from build123d import *

# Parameters (mm, degrees)
SKETCH_1_W               = 38
SKETCH_1_H               = 29
EXTRUDE_1_DEPTH          = 2
SKETCH_2_W               = 2
SKETCH_2_H               = 36
EXTRUDE_2_DEPTH          = 7.5
SKETCH_3_R               = 5
SKETCH_3_R_2             = 1.25
CUT_EXTRUDE_1_DEPTH      = 8.5
CUT_EXTRUDE_1_DEPTH_BACK = 3
SKETCH_4_R               = 1.3
CUT_EXTRUDE_2_DEPTH      = 39
CUT_EXTRUDE_3_DEPTH      = 39
FILLET_1_R               = 2
FILLET_3_R               = 0.5
FILLET_4_R               = 2


with BuildPart() as part:
    # 스케치1 → 보스-돌출1 (new body)
    with BuildSketch(Plane(origin=(0, 0, 0), x_dir=(1, 0, 0), z_dir=(0, 1, 0))):
        with Locations((19, 14.5)):
            Rectangle(SKETCH_1_W, SKETCH_1_H)
    extrude(amount=EXTRUDE_1_DEPTH)

    # 스케치2 → 보스-돌출2 (add)
    with BuildSketch(Plane(origin=(0, 2, 0), x_dir=(1, 0, 0), z_dir=(0, 1, 0))):
        with Locations((1, 18)):
            Rectangle(SKETCH_2_W, SKETCH_2_H)
        with Locations((37, 18)):
            Rectangle(SKETCH_2_W, SKETCH_2_H)
    extrude(amount=EXTRUDE_2_DEPTH)

    # 스케치3 → 컷-돌출1 (cut, two sides)
    with BuildSketch(Plane(origin=(0, 2, 0), x_dir=(1, 0, 0), z_dir=(0, 1, 0))) as cut_extrude_1_sk:
        with Locations((19, 14.5)):
            Circle(SKETCH_3_R)
        with Locations((19, 25.5)):
            Circle(SKETCH_3_R_2)
        with Locations((26.778174593, 22.278174593)):
            Circle(SKETCH_3_R_2)
        with Locations((30, 14.5)):
            Circle(SKETCH_3_R_2)
        with Locations((26.778174593, 6.721825407)):
            Circle(SKETCH_3_R_2)
        with Locations((19, 3.5)):
            Circle(SKETCH_3_R_2)
        with Locations((11.221825407, 6.721825407)):
            Circle(SKETCH_3_R_2)
        with Locations((8, 14.5)):
            Circle(SKETCH_3_R_2)
        with Locations((11.221825407, 22.278174593)):
            Circle(SKETCH_3_R_2)
        with Locations((13, 25.5)):
            Circle(SKETCH_3_R_2)
        with Locations((25, 25.5)):
            Circle(SKETCH_3_R_2)
        with Locations((30, 20.5)):
            Circle(SKETCH_3_R_2)
        with Locations((30, 8.5)):
            Circle(SKETCH_3_R_2)
        with Locations((25, 3.5)):
            Circle(SKETCH_3_R_2)
        with Locations((13, 3.5)):
            Circle(SKETCH_3_R_2)
        with Locations((8, 8.5)):
            Circle(SKETCH_3_R_2)
        with Locations((8, 20.5)):
            Circle(SKETCH_3_R_2)
        with Locations((15.5, 22.278174593)):
            Circle(SKETCH_3_R_2)
        with Locations((22.5, 22.278174593)):
            Circle(SKETCH_3_R_2)
        with Locations((26.778174593, 18)):
            Circle(SKETCH_3_R_2)
        with Locations((26.778174593, 11)):
            Circle(SKETCH_3_R_2)
        with Locations((22.5, 6.721825407)):
            Circle(SKETCH_3_R_2)
        with Locations((15.5, 6.721825407)):
            Circle(SKETCH_3_R_2)
        with Locations((11.221825407, 11)):
            Circle(SKETCH_3_R_2)
        with Locations((11.221825407, 18)):
            Circle(SKETCH_3_R_2)
    extrude(amount=CUT_EXTRUDE_1_DEPTH, mode=Mode.SUBTRACT)
    extrude(cut_extrude_1_sk.sketch, amount=-CUT_EXTRUDE_1_DEPTH_BACK, mode=Mode.SUBTRACT)

    # 스케치4 → 컷-돌출2 (cut, through all)
    with BuildSketch(Plane(origin=(38, 0, 0), x_dir=(0, 0, -1), z_dir=(1, 0, 0))):
        with Locations((3.5, 6.7)):
            Circle(SKETCH_4_R)
        with Locations((25.5, 6.7)):
            Circle(SKETCH_4_R)
        with Locations((10.5, 6.7)):
            Circle(SKETCH_4_R)
        with Locations((32.5, 6.7)):
            Circle(SKETCH_4_R)
    extrude(amount=-CUT_EXTRUDE_2_DEPTH, mode=Mode.SUBTRACT)

    # 스케치5 → 컷-돌출3 (cut, through all)
    with BuildSketch(Plane(origin=(38, 0, 0), x_dir=(0, 0, -1), z_dir=(1, 0, 0))):
        Polygon((36, 3.77094162), (29, 2), (36, 2), align=None)
        Polygon((29, 2), (28.116343093, 0), (29, 0), align=None)
    extrude(amount=-CUT_EXTRUDE_3_DEPTH, mode=Mode.SUBTRACT)

    # 필렛1
    fillet_1_edges = [part.edges().sort_by_distance(p)[0] for p in [
        (1, 9.5, -36),
        (1, 9.5, 0),
        (37, 3.77094162, -36),
        (37, 9.5, 0),
        (37, 9.5, -36),
    ]]
    fillet(fillet_1_edges, radius=FILLET_1_R)

    # 필렛3
    fillet_3_edges = [part.edges().sort_by_distance(p)[0] for p in [
        (2, 2, -14.5),
        (36, 2, -14.5),
    ]]
    fillet(fillet_3_edges, radius=FILLET_3_R)

    # 필렛4
    fillet_4_edges = [part.edges().sort_by_distance(p)[0] for p in [
        (0, 0, -14.058171546),
        (38, 0, -14.058171546),
    ]]
    fillet(fillet_4_edges, radius=FILLET_4_R)


solid = part.part
CAD build for the part. Positions are in the model's coordinates, mm. A direction names the side the tool comes from. Round coordinates to 2 decimals unless told otherwise and drop trailing zeros. Write each loop counter-clockwise with the first axis right and the second up, starting at its lowest first coordinate (ties: lowest second). Pieces come first, ordered by that corner, then holes.
(1) Drop flat-ended pins along their axis: P1, Ø3, axis at x = 14, z = -22, coming from the +Y side; P2, Ø1.5, axis at x = 26.78, z = -22.28, coming from the +Y side; P3, Ø8, axis at x = 33.5, z = -15.5, coming from the +Y side. Give the stop position or say it passes through.
(2) Slice it at C-C, the plane x = 30. Write the cut outline in (y, z).
(3) 3-axis set-ups, long thin cutter, end or side, ignore diameter. For faces 4 (the face through (36.986, 4.085, -35.567)), 5 (the face through (37.014, 5.547, -11.1)): which of +Z, -Z, +X, -X, +Y, -Y reach the whole face in a straight line?
(4) Slice it at A-A, the plane x = 13. Write the cut outline in (y, z).
(5) Probe line 1 along X through (y, z) = (5.5, -17.5); line 2 along X through (y, z) = (1.4, -11); line 3 along X through (y, z) = (1.75, -22). List the from-to ranges inside material, lowest first.
(6) Slice it at D-D, the plane z = -20. Write the cut outline in (x, y), and give its area (3 significant figures).
(7) Mould opens along Z. For faces 1 (the face through (27.45, 1.014, -12.054)), 2 (the face through (15, 2, -18)), 3 (the face through (19.266, 1.014, -28.564)) say: pulls with the +Z half, pulls with the -Z half, needs draft (parallel to the pull), parting line crosses it, or undercut.
(8) Slice it at B-B, the plane z = -25.5. Count the separate pieces of the cut face and the enclosed holes in it, and give its area (3 significant figures).
From the geometry:
1. P1: stops at y = 2
1. P2: passes through
1. P3: stops at y = 9.5
2. outline: (0, -28.12) - (2, -29) - (2, -21.75) - (0, -21.75) - close; (0, -19.25) - (2, -19.25) - (2, -15.75) - (0, -15.75) - close; (0, -13.25) - (2, -13.25) - (2, -9.75) - (0, -9.75) - close; (0, -7.25) - (2, -7.25) - (2, 0) - (0, 0) - close
3. face 4: -Z, +X, -Y
3. face 5: +X, -X
4. outline: (0, -28.12) - (2, -29) - (2, -26.75) - (0, -26.75) - close; (0, -24.25) - (2, -24.25) - (2, -4.75) - (0, -4.75) - close; (0, -2.25) - (2, -2.25) - (2, 0) - (0, 0) - close
5. line 1: x = 0 to 2, 36 to 38
5. line 2: x = 0.09 to 9.97, 12.47 to 15.43, 22.57 to 25.53, 28.03 to 37.91
5. line 3: x = 0.02 to 10, 12.44 to 14.28, 16.72 to 21.28, 23.72 to 25.56, 28 to 37.98
6. outline: (0, 2) arc R2 ccw to (2, 0) - (6.85, 0) - (6.85, 2) - (2.5, 2) arc R0.5 cw to (2, 2.5) - (2, 9.5) - (0, 9.5) - close; (9.15, 0) - (28.85, 0) - (28.85, 2) - (9.15, 2) - close; (31.15, 0) - (36, 0) arc R2 ccw to (38, 2) - (38, 9.5) - (36, 9.5) - (36, 2.5) arc R0.5 cw to (35.5, 2) - (31.15, 2) - close
6. area: 95.2 mm2
7. face 1: undercut
7. face 2: needs draft
7. face 3: pulls with the -Z half
8. separate pieces: 6
8. enclosed holes: 0
8. area: 79.0 mm2
